Source: CAD feature listing. Evaluate the final solid. Frame: model axes, mm. A direction names the side the tool comes from. Give positions to 0.01 mm unless a question says otherwise; leave off trailing zeros. Loops run counter-clockwise (first coordinate to the right, second up) from the corner with the lowest first, then second, coordinate; pieces in that order, holes last. Notation, with made-up numbers: (52, 14) - (73, 14) arc R17 ccw to (73, 46) - close; hole circle Ø7 at (12.5, 36.25). An arc over 180 degrees is marked (long way). Put each result on its own line as item: value.
```python
from build123d import *

# Parameters (mm, degrees)
F0_R     = 9.92251
F1_DEPTH = 7.9375
F2_W     = 57.15
F2_H     = 36.5125
F3_DEPTH = 7.9375
F5_R     = 10.3251
F6_DEPTH = 7.9375
F7_R     = 4.7625


with BuildPart() as f1:
    # F0 (on Front) → F1 (new body)
    with BuildSketch(Plane.XZ):
        with BuildLine():
            Line((0, 44.45), (0, 0))
            Line((0, 0), (57.15, 0))
            Line((57.15, 0), (57.15, 44.45))
            ThreePointArc((57.15, 44.45), (28.575, 73.025), (0, 44.45))
        make_face()
        with Locations((28.575, 44.45)):
            Circle(F0_R, mode=Mode.SUBTRACT)
    extrude(amount=F1_DEPTH)

    # F2 (on Top) → F3 (join)
    with BuildSketch(Plane.XY):
        with Locations((28.575, 18.25625)):
            Rectangle(F2_W, F2_H)
    extrude(amount=F3_DEPTH)

    # F4: F1 across face


with BuildPart() as f1_1:
    add(f1.part)
    add(f1.part.mirror(Plane(origin=(28.575, 36.5125, 3.96875), x_dir=(-1, 0, 0), z_dir=(0, 1, 0))))

    # F5 (on Top) → F6 (join)
    with BuildSketch(Plane.XY):
        with BuildLine():
            Line((57.15, 58.7375), (57.15, 14.2875))
            Line((57.15, 14.2875), (111.125, 14.2875))
            ThreePointArc((111.125, 14.2875), (133.35, 36.5125), (111.125, 58.7375))
            Line((111.125, 58.7375), (57.15, 58.7375))
        make_face()
        with Locations((73.025, 36.5125)):
            Circle(F5_R, mode=Mode.SUBTRACT)
        with Locations((111.125, 36.5125)):
            Circle(F5_R, mode=Mode.SUBTRACT)
    extrude(amount=F6_DEPTH)

    # F7
    f7_edges = [f1_1.edges().sort_by_distance(p)[0] for p in [
        (28.575, 73.025, 7.9375),
        (28.575, 0, 7.9375),
        (28.575, -7.9375, 0),
        (28.575, 80.9625, 0),
    ]]
    fillet(f7_edges, radius=F7_R)


solid = f1_1.part
```
1) Section query C-C, the plane x = 20.5. Output: boundary loops of the cut face in (y, z) (1 decimal).
Check result:
outline: (-7.9, 4.8) arc R4.8 ccw to (-3.2, 0) - (76.2, 0) arc R4.8 ccw to (81, 4.8) - (81, 38.7) - (73, 38.7) - (73, 12.7) arc R4.8 cw to (68.3, 7.9) - (4.8, 7.9) arc R4.8 cw to (0, 12.7) - (0, 38.7) - (-7.9, 38.7) - close; (-7.9, 50.2) - (0, 50.2) - (0, 71.9) - (-7.9, 71.9) - close; (73, 50.2) - (81, 50.2) - (81, 71.9) - (73, 71.9) - close
2) Access query for faces 5 (the flat face through (57.15, 75, 17)), 6 (the flat face through (51, 36, 7.938)), 7 (the flat face through (51, 36, 0)), 8 (the flat face through (57.15, -2, 17)). Directions: +Z, -Z, +X, -X, +Y, -Y. A direction counts if a zero-diameter tool reaches every point of the face in a straight line with its end or side. Return the directions, or none.
Check result:
face 5: +Z, -Z, +X, +Y
face 6: +Z, +X, -X
face 7: -Z, +X, -X, +Y, -Y
face 8: +Z, -Z, +X, -Y
3) Section query B-B, the plane x = 68. Output: boundary loops of the cut face in (y, z), plus the area to 3 significant figures.
Check result:
outline: (14.29, 0) - (27.49, 0) - (27.49, 7.94) - (14.29, 7.94) - close; (45.53, 0) - (58.74, 0) - (58.74, 7.94) - (45.53, 7.94) - close
area: 210 mm²
4) Pin query (flat end, axial travel): P1, Ø5, axis at x = 64, z = 9.5, coming from the -Y side; P2, Ø11, axis at y = -1, z = 24.5, coming from the +X side; P3, Ø19, axis at x = 89, y = 45.5, coming from the +Z side. Return the tip coordinate at first contact, or that it passes through.
Check result:
P1: y = 14.29
P2: x = 57.15
P3: z = 7.94
5) Section query D-D, the plane z = 42. State how many separate pieces and enclosed holes the cut face has, plus the area to 3 significant figures.
Check result:
separate pieces: 4
enclosed holes: 0
area: 602 mm²
6) Mould query, pull axis X, two halves, no side actions, for faces 1 (the cylindrical face through (64.83, 30.23, 3.91)), 2 (the flat face through (0, 37, 7)), 3 (the cylindrical face through (120.973, 39.614, 3.913)), 4 (the flat face through (85, 58.738, 4)). Classes: pulls with the +X half, pulls with the -X half, needs draft (parallel to the pull), parting line crosses it, or undercut.
Check result:
face 1: undercut
face 2: pulls with the -X half
face 3: undercut
face 4: needs draft
7) Material intervals for line 1 along Y through (x, z) = (35, 27) (1 decimal); line 2 along X through (y, z) = (78, 44); line 3 along Z through (x, y) = (6, 14), sorted ascending. Write a range as [from, to].
Check result:
line 1: [-7.9, 0], [73, 81]
line 2: [0, 18.66], [38.49, 57.15]
line 3: [0, 7.94]
